```python
from build123d import *

# Parameters (mm, degrees)
SKETCH1_W           = 25
SKETCH1_H           = 70
BOSS_EXTRUDE1_DEPTH = 4
BOSS_EXTRUDE2_DEPTH = 5
BOSS_EXTRUDE3_DEPTH = 5
SKETCH5_W           = 7
SKETCH5_H           = 60
SKETCH5_R           = 1.5
BOSS_EXTRUDE4_DEPTH = 5
CUT_EXTRUDE1_REACH  = 43.785
SKETCH6_W           = 2
SKETCH6_H           = 25


with BuildPart() as part:
    # Sketch1 → Boss-Extrude1 (new body)
    with BuildSketch(Plane.XY):
        Rectangle(SKETCH1_W, SKETCH1_H)
    extrude(amount=BOSS_EXTRUDE1_DEPTH)

    # Sketch2 → Boss-Extrude2 (add)
    with BuildSketch(Plane(origin=(0, 35, 0), x_dir=(1, 0, 0), z_dir=(0, 1, 0))):
        Polygon((-4.787407973, -6), (-10.5, -10), (-12.5, -10), (-12.5, -4), (12.5, -4), (12.5, -11), (2.353332061, -11), align=None)
    extrude(amount=-BOSS_EXTRUDE2_DEPTH)

    # Sketch3 → Boss-Extrude3 (add)
    with BuildSketch(Plane.XZ.offset(35)):
        Polygon((2.353332061, 11), (-4.787407973, 6), (-10.5, 10), (-12.5, 10), (-12.5, 4), (12.5, 4), (12.5, 11), align=None)
    extrude(amount=-BOSS_EXTRUDE3_DEPTH)

    # Sketch5 → Boss-Extrude4 (add)
    with BuildSketch(Plane(origin=(12.5, 0, 0), x_dir=(0, 0, -1), z_dir=(1, 0, 0))):
        with Locations((-7.5, 0)):
            Rectangle(SKETCH5_W, SKETCH5_H)
        with Locations((-7, 18)):
            Circle(SKETCH5_R, mode=Mode.SUBTRACT)
        with Locations((-7, -18)):
            Circle(SKETCH5_R, mode=Mode.SUBTRACT)
    extrude(amount=-BOSS_EXTRUDE4_DEPTH)

    # Sketch6 → Cut-Extrude1 (cut, up to next)
    with BuildSketch(Plane.ZY.offset(-7.5), mode=Mode.PRIVATE) as cut_extrude1_sk1:
        with Locations((10, 0)):
            Rectangle(SKETCH6_W, SKETCH6_H)
    cut_extrude1_tool1 = extrude(cut_extrude1_sk1.sketch, amount=-CUT_EXTRUDE1_REACH, mode=Mode.PRIVATE) & part.part
    add(cut_extrude1_tool1.solids().sort_by_distance((7.5, 0, 10))[0], mode=Mode.SUBTRACT)


solid = part.part
```
Build history of the part. All positions in model axes, mm. A direction names the side the tool comes from. Coordinates: 2 decimals unless noted, no trailing zeros. Order: outer loops, then holes, each group sorted by start corner. A loop starts at its lowest first (then second) coordinate and runs counter-clockwise, first axis right, second up.
Item 1: Saw through at B-B on z = 4.75. List the corners of the cut face in (x, y), then the cut area to 3 significant figures.
Filled in:
outline: (-12.5, -35) - (12.5, -35) - (12.5, 35) - (-12.5, 35) - (-12.5, 30) - (7.5, 30) - (7.5, -30) - (-12.5, -30) - close
area: 550 mm2
Item 2: Saw through at C-C on x = 4.5. List the corners of the cut face in (y, z), then the cut area to 3 significant figures.
Filled in:
outline: (-35, 0) - (35, 0) - (35, 11) - (30, 11) - (30, 4) - (-30, 4) - (-30, 11) - (-35, 11) - close
area: 350 mm2
Item 3: Tool access for faces 4 (the flat face through (7.5, 0, 8)), 5 (the flat face through (0, -35, 4)), 6 (the flat face through (10, 0, 9)), 7 (the flat face through (-11, -33, 10)), 8 (the flat face through (-7.6, -32.53, 7.97)): list every direction of +Z, -Z, +X, -X, +Y, -Y with a clear straight run to the whole face (end or side of a thin tool).
Filled in:
face 4: +Z, -X
face 5: +Z, -Z, +X, -X, -Y
face 6: +Z, +X, -X
face 7: +Z, -X, +Y, -Y
face 8: +Z, +Y, -Y
Item 4: Mould opens along Y. For faces 1 (the flat face through (12.5, 0, 6)), 2 (the flat face through (10, 12.5, 10)), 3 (the flat face through (0, 35, 5)) say: released by +Y, released by -Y, zero draft, split by the parting line, or undercut.
Filled in:
face 1: zero draft
face 2: undercut
face 3: released by +Y
Item 5: Saw through at A-A on y = -18. List the corners of the cut face in (x, z), then the cut area to 3 significant figures.
Filled in:
outline: (-12.5, 0) - (12.5, 0) - (12.5, 5.5) - (7.5, 5.5) - (7.5, 4) - (-12.5, 4) - close; (7.5, 8.5) - (12.5, 8.5) - (12.5, 11) - (7.5, 11) - close
area: 120 mm2
Item 6: Drill centre lines: L1, parallel to Y at x = 9.4, z = 7; L2, parallel to Y at x = -8.5, z = 5.25; L3, parallel to Z at x = 8.5, y = 1. Where is each one in solid material? Low to high.
Filled in:
L1: y = -35 to -19.5, -16.5 to 16.5, 19.5 to 35
L2: y = -35 to -30, 30 to 35
L3: z = 0 to 9
Item 7: Drop flat-ended pins along their axis: pin 1 Ø2.5 at (y, z) = (-18, 7) entering from -X; pin 2 Ø1 at (x, y) = (-10, 4.5) entering from +Z; pin 3 Ø0.6 at (x, y) = (-11.5, -33) entering from +Z; pin 4 Ø4 at (y, z) = (18, 7) entering from -X. Give the stop position or say it passes through.
Filled in:
pin 1: passes through
pin 2: stops at z = 4
pin 3: stops at z = 10
pin 4: stops at x = 7.5
Item 8: Saw through at D-D on y = 14. List the corners of the cut face in (x, z), then the cut area to 3 significant figures.
Filled in:
outline: (-12.5, 0) - (12.5, 0) - (12.5, 11) - (7.5, 11) - (7.5, 4) - (-12.5, 4) - close
area: 135 mm2
